from build123d import *

# Parameters (mm, degrees)
F0_W     = 25.4
F0_H     = 4.7625
F0_H_2   = 19.05
F1_DEPTH = 12.7


with BuildPart() as f1:
    # F0 (on Front) → F1 (new body, symmetric)
    with BuildSketch(Plane.XZ):
        Polygon((41.275, -9.525), (41.275, 9.525), (22.225, 9.525), (-41.275, 9.525), (-41.275, -9.525), align=None)
        with BuildLine():
            Line((22.225, 9.525), (41.275, 9.525))
            Line((41.275, 9.525), (41.275, 26.9875))
            ThreePointArc((41.275, 26.9875), (45.9246798487, 38.2128201513), (57.15, 42.8625))
            Line((57.15, 42.8625), (60.325, 42.8625))
            Line((60.325, 42.8625), (60.325, 61.9125))
            Line((60.325, 61.9125), (57.15, 61.9125))
            add(Edge.make_bspline(
                [(56.6181319004, 61.9084498915), (56.7953297588, 61.9100229776), (56.9726195791, 61.9113731218), (57.15, 61.9125)],
                knots=[111.1262909872, 111.1262909872, 111.1262909872, 111.1262909872, 111.4985685166, 111.4985685166, 111.4985685166, 111.4985685166], degree=3))
            ThreePointArc((56.6181319004, 61.9084498915), (32.2669624204, 51.4944391359), (22.225, 26.9875))
            Line((22.225, 26.9875), (22.225, 9.525))
        make_face()
        with BuildLine():
            Line((-41.275, 9.525), (22.225, 9.525))
            Line((22.225, 9.525), (22.225, 26.9875))
            ThreePointArc((22.225, 26.9875), (32.2669624204, 51.4944391359), (56.6181319004, 61.9084498915))
            add(Edge.make_bspline(
                [(-41.275, 9.525), (-40.9761398409, 41.1041646748), (3.723881742, 61.4388775764), (56.6181319004, 61.9084498915)],
                knots=[0, 0, 0, 0, 111.1262909872, 111.1262909872, 111.1262909872, 111.1262909872], degree=3))
        make_face()
        with BuildLine():
            ThreePointArc((57.15, 61.9125), (56.8840582401, 61.9114874582), (56.6181319004, 61.9084498915))
            add(Edge.make_bspline(
                [(56.6181319004, 61.9084498915), (56.7953297588, 61.9100229776), (56.9726195791, 61.9113731218), (57.15, 61.9125)],
                knots=[111.1262909872, 111.1262909872, 111.1262909872, 111.1262909872, 111.4985685166, 111.4985685166, 111.4985685166, 111.4985685166], degree=3))
        make_face()
        with Locations((73.025, 40.48125)):
            Rectangle(F0_W, F0_H)
        with Locations((73.025, 52.3875)):
            Rectangle(F0_W, F0_H_2)
        with Locations((73.025, 64.29375)):
            Rectangle(F0_W, F0_H)
        Polygon((85.725, 61.9125), (85.725, 42.8625), (85.725, 38.1), (111.125, 38.1), (111.125, 66.675), (85.725, 66.675), align=None)
    extrude(amount=F1_DEPTH, both=True)


solid = f1.part
Part model, mm, in its own coordinate system. A direction names the side the tool comes from. Coordinates: 2 decimals unless noted, no trailing zeros. Loops run counter-clockwise (first coordinate to the right, second up) from the corner with the lowest first, then second, coordinate; pieces in that order, holes last. Notation, with made-up numbers: M 16,19 L 21,19 A24 cw 21,53 Z; hole C -35.5,7 d7. An arc over 180 degrees is marked long. Use a Markdown table: item, result. Add a question column.
Q1. Mould opens along X. For faces 4 (the flat face through (-41.275, 0, 0)), 5 (the flat face through (59, 0, 61.912)), 6 (the cylindrical face through (45.802, -0.178, 38.089)) say: +X half, -X half, draft (parallel to the pull), parting line (faces both ways), or undercut.
Q2. Pin check, flat tips, straight feed: P1, Ø12, axis at x = 50, z = 38, coming from the +Y side; P2, Ø2.5, axis at x = 58.5, y = 1, coming from the +Z side; P3, Ø12.5, axis at y = 3.5, z = 6.5, coming from the +X side (3 decimals); P4, Ø3, axis at x = 86.5, y = -8.5, coming from the -Z side. Stop position of each tip, or through.
Q3. Probe L1, parallel to X at y = -1.5, z = 2 (3 decimals); L2, parallel to Z at x = 75, y = 5.75 (3 decimals); L3, parallel to Z at x = 60, y = -6. List the from-to ranges inside material, lowest first.
Q4. Cut at A-A (x = 87). Write the cut outline in (y, z) (3 decimals), and give its area (3 significant figures).
Q5. Which spindle directions (+Z, -Z, +X, -X, +Y, -Y) get a long thin tool onto all of the face, cutting with end or side? Do faces 1 (the flat face through (60.325, 0, 64)), 2 (the flat face through (60.325, 0, 40)), 3 (the flat face through (85, 0, 38.1)). Say none if no direction does.
Worked out:
| question | item | result |
|---|---|---|
| 1 | face 4 | -X half |
| 1 | face 5 | draft |
| 1 | face 6 | undercut |
| 2 | P1 | stops at y = 12.7 |
| 2 | P2 | stops at z = 61.91 |
| 2 | P3 | stops at x = 41.275 |
| 2 | P4 | stops at z = 38.1 |
| 3 | L1 | x = -41.275 to 41.275 |
| 3 | L2 | z = 38.1 to 66.675 |
| 3 | L3 | z = 42.86 to 61.91 |
| 4 | outline | M -12.7,38.1 L 12.7,38.1 L 12.7,66.675 L -12.7,66.675 Z |
| 4 | area | 726 mm2 |
| 5 | face 1 | +Z, -X, +Y, -Y |
| 5 | face 2 | -Z, +Y, -Y |
| 5 | face 3 | -Z, +X, +Y, -Y |
